The listing builds one solid part. Answer for the finished solid, in the listing's coordinates (mm). A direction names the side the tool comes from. Round coordinates to 2 decimals unless told otherwise and drop trailing zeros. Use CSV: the item, a comma, the result in double quotes. Start each with the question number.
Item 1: Straight lines are drawn through the part: line 1 along Z through (x, y) = (13, 71) (3 decimals); line 2 along Y through (x, z) = (-62, 33); line 3 along Y through (x, z) = (-56, 15.5). For each, find the intervals that lie inside material, in ascending order. Write a range as [from, to].
Item 2: Determine the mould class of faces 1 (the flat face through (-88.106, 72, -9)), 2 (the flat face through (-1, -9, -38.1)), 3 (the flat face through (18, 72, -22.225)) for opening direction X: +X half, -X half, draft (parallel to the pull), parting line (faces both ways), or undercut.
Item 3: Flat-ended cylindrical pins translate along their axes: P1, Ø0.8, axis at x = -70, y = 80, coming from the +Z side; P2, Ø9, axis at y = 76, z = 24, coming from the +X side; P3, Ø5, axis at x = 23.5, y = 70, coming from the -Z side (3 decimals). Find the tip coordinate at first contact, or state that the pin passes through.
Item 4: Find section A-A, the plane z = -31.5. Count the separate pieces of the cut face and the enclosed holes in it, plus the area to 3 significant figures.
Item 5: For faces 4 (the flat face through (-70.644, 77, 25)), 5 (the flat face through (18, 62.706, -29)), 6 (the flat face through (-19, 62.706, 29)), 7 (the flat face through (69.056, 77, 25)), determine the directions among +Z, -Z, +X, -X, +Y, -Y from which every point of the face is accessible in a straight line to the end or side of a thin tool.
```python
from build123d import *

# Parameters (mm, degrees)
SKETCH1_W          = 179.3875
SKETCH1_H          = 166.6875
EXTRUDE1_DEPTH     = 38.1
SKETCH2_W          = 179.3875
SKETCH2_H          = 76.2
SKETCH2_W_2        = 176.2125
SKETCH2_H_2        = 73.025
CUT_EXTRUDE1_DEPTH = 22.225
SKETCH3_W          = 47.625
SKETCH3_H          = 20.6375
CUT_EXTRUDE2_DEPTH = 12.7
SKETCH4_W          = 35.71875
SKETCH4_H          = 17.4625
CUT_EXTRUDE3_DEPTH = 14.2875
FILLET1_R          = 1.5748
FILLET2_R          = 3.175
SKETCH5_W          = 1.5875
SKETCH5_H          = 11.1125
EXTRUDE3_DEPTH     = 12.7


with BuildPart() as part:
    # Sketch1 → Extrude1 (new, symmetric)
    with BuildSketch(Plane.XY):
        Rectangle(SKETCH1_W, SKETCH1_H)
    extrude(amount=EXTRUDE1_DEPTH, both=True)

    # Sketch2 → Cut-Extrude1 (cut)
    with BuildSketch(Plane(origin=(0, 83.34375, 0), x_dir=(-1, 0, 0), z_dir=(0, 1, 0))):
        Rectangle(SKETCH2_W, SKETCH2_H)
        Rectangle(SKETCH2_W_2, SKETCH2_H_2, mode=Mode.SUBTRACT)
    extrude(amount=-CUT_EXTRUDE1_DEPTH, mode=Mode.SUBTRACT)

    # Sketch3 → Cut-Extrude2 (cut)
    with BuildSketch(Plane(origin=(0, 83.34375, 0), x_dir=(-1, 0, 0), z_dir=(0, 1, 0))):
        with Locations((-64.29375, 26.19375)):
            Rectangle(SKETCH3_W, SKETCH3_H)
        with Locations((64.29375, 26.19375)):
            Rectangle(SKETCH3_W, SKETCH3_H)
    extrude(amount=-CUT_EXTRUDE2_DEPTH, mode=Mode.SUBTRACT)

    # Sketch4 → Cut-Extrude3 (cut)
    with BuildSketch(Plane.XY.offset(36.5125)):
        with Locations((-18.653125, 71.4375)):
            Rectangle(SKETCH4_W, SKETCH4_H)
        with Locations((18.653125, 71.4375)):
            Rectangle(SKETCH4_W, SKETCH4_H)
    cut_extrude3 = extrude(amount=-CUT_EXTRUDE3_DEPTH, mode=Mode.SUBTRACT)

    # Mirror1: Cut-Extrude3 across plane
    add(cut_extrude3.mirror(Plane.XY), mode=Mode.SUBTRACT)

    # Fillet1
    fillet1_edges = [part.edges().sort_by_distance(p)[0] for p in [
        (89.69375, 61.11875, 0),
        (0, 61.11875, 38.1),
        (-89.69375, 61.11875, 0),
        (0, 61.11875, -38.1),
        (0, 83.34375, -36.5125),
        (-88.10625, 83.34375, -10.31875),
        (88.10625, 83.34375, -10.31875),
        (88.10625, 70.64375, 26.19375),
        (88.10625, 76.99375, 15.875),
        (64.29375, 70.64375, 36.5125),
        (40.48125, 70.64375, 26.19375),
        (40.48125, 76.99375, 36.5125),
        (64.29375, 70.64375, 15.875),
        (64.29375, 83.34375, 15.875),
        (40.48125, 83.34375, 26.19375),
        (0, 83.34375, 36.5125),
        (-88.10625, 70.64375, 26.19375),
        (-64.29375, 70.64375, 15.875),
        (-88.10625, 76.99375, 15.875),
        (-40.48125, 70.64375, 26.19375),
        (-64.29375, 70.64375, 36.5125),
        (-40.48125, 76.99375, 36.5125),
        (-40.48125, 83.34375, 26.19375),
        (-64.29375, 83.34375, 15.875),
    ]]
    fillet(fillet1_edges, radius=FILLET1_R)

    # Fillet2
    # the kernel refuses this fillet: 3.175 mm, written as the material it takes off along each edge
    with BuildSketch(Plane(origin=(-86.51875, -80.16875, -34.925), x_dir=(-1, 0, 0), z_dir=(0, 0, -1))) as fillet2_piece_1_section:
        Polygon((0, 0), (FILLET2_R * 1.02, 0), (FILLET2_R * 1.02, -FILLET2_R * 1.02), (0, -FILLET2_R * 1.02), align=None)
    fillet2_piece_1 = extrude(amount=FILLET2_R * 1.02, mode=Mode.PRIVATE)
    fillet2_piece_1 = fillet2_piece_1 - Plane(origin=(-86.51875, -80.16875, -34.925), x_dir=(0.7071067811865475, 0.7071067811865477, 0), z_dir=(0, 0, -1)) * Sphere(FILLET2_R, mode=Mode.PRIVATE)
    add(fillet2_piece_1, mode=Mode.SUBTRACT)
    with BuildSketch(Plane(origin=(-86.51875, -80.16875, 34.925), x_dir=(-1, 0, 0), z_dir=(0, 0, 1))) as fillet2_piece_2_section:
        Polygon((0, 0), (FILLET2_R * 1.02, 0), (FILLET2_R * 1.02, FILLET2_R * 1.02), (0, FILLET2_R * 1.02), align=None)
    fillet2_piece_2 = extrude(amount=FILLET2_R * 1.02, mode=Mode.PRIVATE)
    fillet2_piece_2 = fillet2_piece_2 - Plane(origin=(-86.51875, -80.16875, 34.925), x_dir=(0.7071067811865475, 0.7071067811865477, 0), z_dir=(0, 0, 1)) * Sphere(FILLET2_R, mode=Mode.PRIVATE)
    add(fillet2_piece_2, mode=Mode.SUBTRACT)
    with BuildSketch(Plane(origin=(86.51875, -80.16875, 34.925), x_dir=(0, 0, 1), z_dir=(1, 0, 0))) as fillet2_piece_3_section:
        Polygon((0, 0), (FILLET2_R * 1.02, 0), (FILLET2_R * 1.02, FILLET2_R * 1.02), (0, FILLET2_R * 1.02), align=None)
    fillet2_piece_3 = extrude(amount=FILLET2_R * 1.02, mode=Mode.PRIVATE)
    fillet2_piece_3 = fillet2_piece_3 - Plane(origin=(86.51875, -80.16875, 34.925), x_dir=(0, 0.7071067811865475, -0.7071067811865475), z_dir=(1, 0, 0)) * Sphere(FILLET2_R, mode=Mode.PRIVATE)
    add(fillet2_piece_3, mode=Mode.SUBTRACT)
    with BuildSketch(Plane(origin=(86.51875, -80.16875, -34.925), x_dir=(0, 0, -1), z_dir=(1, 0, 0))) as fillet2_piece_4_section:
        Polygon((0, 0), (FILLET2_R * 1.02, 0), (FILLET2_R * 1.02, -FILLET2_R * 1.02), (0, -FILLET2_R * 1.02), align=None)
    fillet2_piece_4 = extrude(amount=FILLET2_R * 1.02, mode=Mode.PRIVATE)
    fillet2_piece_4 = fillet2_piece_4 - Plane(origin=(86.51875, -80.16875, -34.925), x_dir=(0, 0.7071067811865475, 0.7071067811865475), z_dir=(1, 0, 0)) * Sphere(FILLET2_R, mode=Mode.PRIVATE)
    add(fillet2_piece_4, mode=Mode.SUBTRACT)
    with BuildSketch(Plane(origin=(-89.69375, -83.34375, -34.925), x_dir=(0, 1, 0), z_dir=(0, 0, 1)), Plane(origin=(89.69375, -83.34375, 34.925), x_dir=(0, 1, 0), z_dir=(0, 0, -1))) as fillet2_piece_5:
        with BuildLine():
            CenterArc((FILLET2_R, -FILLET2_R), FILLET2_R, 90, 90)
            Line((0, -FILLET2_R), (0, 0))
            Line((0, 0), (FILLET2_R, 0))
        make_face()
    extrude(amount=69.85, mode=Mode.SUBTRACT)
    with BuildSketch(Plane(origin=(86.51875, -83.34375, 38.1), x_dir=(0, 1, 0), z_dir=(-1, 0, 0))) as fillet2_piece_6:
        with BuildLine():
            CenterArc((FILLET2_R, FILLET2_R), FILLET2_R, 180, 90)
            Line((0, FILLET2_R), (0, 0))
            Line((0, 0), (FILLET2_R, 0))
        make_face()
    extrude(amount=173.0375, mode=Mode.SUBTRACT)
    with BuildSketch(Plane(origin=(86.51875, -83.34375, -38.1), x_dir=(0, 1, 0), z_dir=(-1, 0, 0))) as fillet2_piece_7:
        with BuildLine():
            CenterArc((FILLET2_R, -FILLET2_R), FILLET2_R, 90, 90)
            Line((0, -FILLET2_R), (0, 0))
            Line((0, 0), (FILLET2_R, 0))
        make_face()
    extrude(amount=173.0375, mode=Mode.SUBTRACT)
    with BuildSketch(Plane(origin=(-89.69375, -80.16875, 38.1), x_dir=(1, 0, 0), z_dir=(0, 1, 0)), Plane(origin=(89.69375, 67.48145, -38.1), x_dir=(0, 0, 1), z_dir=(0, -1, 0))) as fillet2_piece_8:
        with BuildLine():
            CenterArc((FILLET2_R, FILLET2_R), FILLET2_R, 180, 90)
            Line((0, FILLET2_R), (0, 0))
            Line((0, 0), (FILLET2_R, 0))
        make_face()
    extrude(amount=147.6502, mode=Mode.SUBTRACT)
    with BuildSketch(Plane(origin=(-89.69375, -80.16875, -38.1), x_dir=(1, 0, 0), z_dir=(0, 1, 0)), Plane(origin=(89.69375, 67.48145, 38.1), x_dir=(0, 0, -1), z_dir=(0, -1, 0))) as fillet2_piece_9:
        with BuildLine():
            CenterArc((FILLET2_R, -FILLET2_R), FILLET2_R, 90, 90)
            Line((0, -FILLET2_R), (0, 0))
            Line((0, 0), (FILLET2_R, 0))
        make_face()
    extrude(amount=147.6502, mode=Mode.SUBTRACT)

    # Sketch5 → Extrude3 (add)
    with BuildSketch(Plane(origin=(0, 70.64375, 0), x_dir=(-1, 0, 0), z_dir=(0, 1, 0))):
        with Locations((-69.85, 24.60625)):
            Rectangle(SKETCH5_W, SKETCH5_H)
        with Locations((69.85, 24.60625)):
            Rectangle(SKETCH5_W, SKETCH5_H)
    extrude(amount=EXTRUDE3_DEPTH)


solid = part.part
```
Worked out:
1,line 1,"z = [-22.225, 22.225]"
1,line 2,"y = [-83.34, 70.64]"
1,line 3,"y = [-83.34, 82.79]"
2,face 1,"-X half"
2,face 2,"draft"
2,face 3,"undercut"
3,P1,"stops at z = 30.16"
3,P2,"stops at x = 70.64"
3,P3,"stops at z = -22.225"
4,separate pieces,"1"
4,enclosed holes,"2"
4,area,"28,600 mm²"
5,face 4,"+Z, -X, +Y"
5,face 5,"-Z"
5,face 6,"+Z"
5,face 7,"+Z, +Y"
